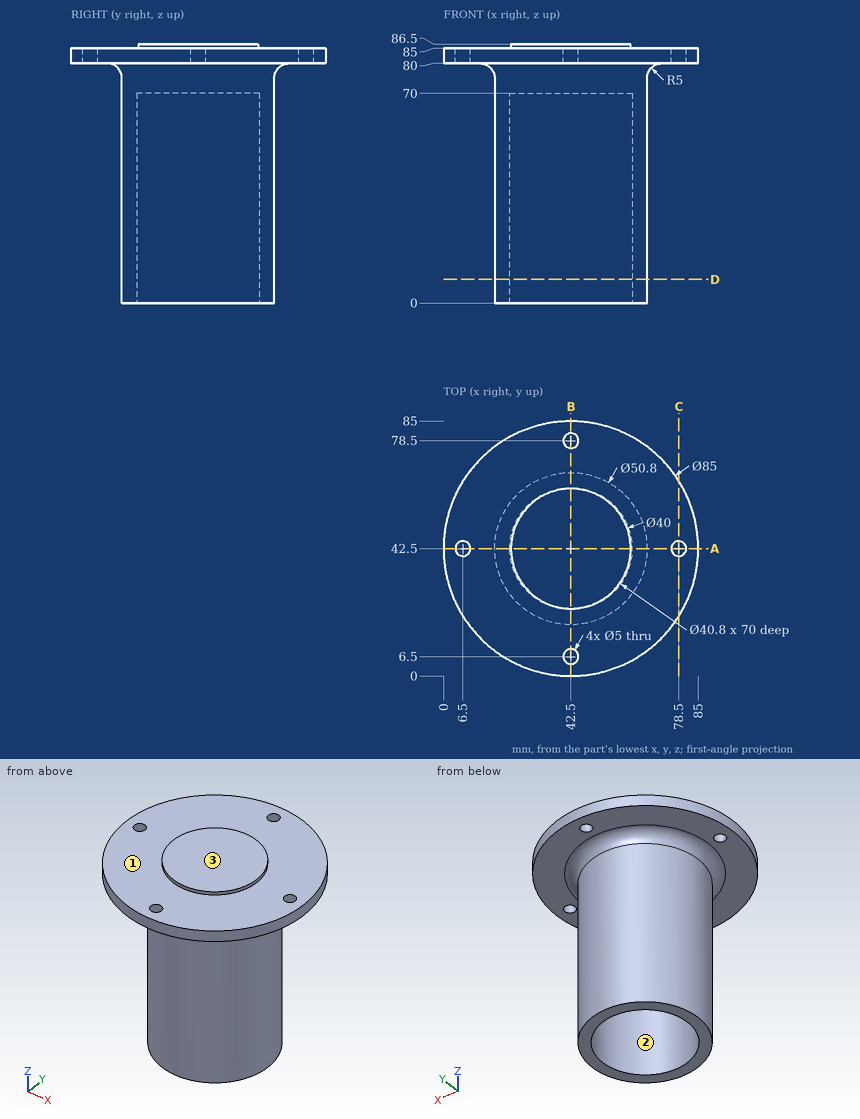
Can you work these out from the drawing? Everything is in mm from the part's minimum corner. A direction names the side the tool comes from. Round coordinates to 2 decimals unless told otherwise and drop trailing zeros. Loops run counter-clockwise (first coordinate to the right, second up) from the corner with the lowest first, then second, coordinate; pieces in that order, holes last. Notation, with made-up numbers: (-4.75, 51) - (26.25, 51) arc R7 cw to (26.25, 55) - close; hole circle Ø1 at (68.25, 44). An arc over 180 degrees is marked (long way). Write item = value, one per line. Start each with the question number.
(1) For the marked faces 1, 2 and 3, which set-ups out of +Z, -Z, +X, -X, +Y, -Y let a thin tool reach every point of the face, with its end or its side?
(2) If we section it at C-C (x = 78.5): Please give me the cut outline in (y, z).
(3) For P1, Ø12, axis at x = 49.5, z = 13, coming from the -Y side; P2, Ø10, axis at x = 62, z = 17, coming from the -Y side; P3, Ø4, axis at x = 78.5, y = 42.5, coming from the +Z side; P4, Ø20.5, axis at x = 47, y = 43, coming from the -Z side, each with a flat end and sliding along its axis, tell me the tip position at first contact or that it passes through.
(4) If we section it at D-D (z = 8): Please give me the cut outline in (x, y).
(5) If we section it at A-A (y = 42.5): Please give me the cut outline in (x, z), and give its area (3 significant figures).
(6) If I drill on probe 1 along Y at (x, z) = (42.5, 81.6); probe 2 along Y at (x, z) = (42, 81); probe 3 along Y at (x, z) = (43.5, 37.5), over which ranges is the centre line in solid material (lowest first)? Write a range as [from, to].
Ans:
q1.face_1 = +Z
q1.face_2 = -Z
q1.face_3 = +Z, +X, -X, +Y, -Y
q2.outline = (19.91, 80) - (40, 80) - (40, 85) - (19.91, 85) - close; (45, 80) - (65.09, 80) - (65.09, 85) - (45, 85) - close
q3.P1 = 17.12
q3.P2 = 21.65
q3.P3 = through
q3.P4 = 70
q4.outline = circle Ø50.8 at (42.5, 42.5); hole circle Ø40.8 at (42.5, 42.5)
q5.outline = (0, 80) - (4, 80) - (4, 85) - (0, 85) - close; (9, 80) - (12.1, 80) arc R5 cw to (17.1, 75) - (17.1, 0) - (22.1, 0) - (22.1, 70) - (62.9, 70) - (62.9, 0) - (67.9, 0) - (67.9, 75) arc R5 cw to (72.9, 80) - (76, 80) - (76, 85) - (62.5, 85) - (62.5, 86.5) - (22.5, 86.5) - (22.5, 85) - (9, 85) - close; (81, 80) - (85, 80) - (85, 85) - (81, 85) - close
q5.area = 1,650 mm²
q6.probe_1 = [0, 4], [9, 76], [81, 85]
q6.probe_2 = [0, 4.05], [8.95, 76.05], [80.95, 85]
q6.probe_3 = [17.12, 22.12], [62.88, 67.88]
